```python
from build123d import *

# Parameters (mm, degrees)
BOSS_EXTRUDE1_DEPTH     = 152.4
CUT_EXTRUDE1_DEPTH      = 1634.518215387
CUT_EXTRUDE1_DEPTH_BACK = 1634.518215387
CUT_EXTRUDE2_DEPTH      = 1634.518215536
FILLET1_R               = 50.8
CUT_EXTRUDE3_DEPTH      = 48.26
CUT_EXTRUDE4_DEPTH      = 1213.010253568
SKETCH6_W               = 101.6
SKETCH6_H               = 127
CUT_EXTRUDE5_DEPTH      = 25.4
LPATTERN1_COUNT         = 2
LPATTERN1_PITCH         = 254
SKETCH7_W               = 304.8
SKETCH7_H               = 127
CUT_EXTRUDE7_DEPTH      = 114.3


with BuildPart() as part:
    # Sketch1 → Boss-Extrude1 (new body)
    with BuildSketch(Plane.XY):
        with BuildLine():
            Line((0, 0), (0, 381))
            Line((0, 381), (457.2, 1016))
            Line((457.2, 1016), (1270, 1016))
            Line((1270, 1016), (1270, 381))
            ThreePointArc((1270, 381), (1000.592316368, 269.407683632), (889, 0))
            Line((889, 0), (0, 0))
        make_face()
    extrude(amount=BOSS_EXTRUDE1_DEPTH)

    # Sketch3 → Cut-Extrude1 (cut, two sides: drawn at the far end of the back side and taken through both)
    with BuildSketch(Plane(origin=(1270, 0, 0), x_dir=(0, 0, -1), z_dir=(1, 0, 0)).offset(-CUT_EXTRUDE1_DEPTH_BACK)):
        with BuildLine():
            Line((0, 1016), (-114.3, 1016))
            add(Edge.make_bspline(
                [(-114.3, 1016), (-8.40924149, 829.104015067), (-15.870449407, 600.128785321), (0, 381)],
                knots=[0, 0, 0, 0, 1, 1, 1, 1], degree=3))
            Line((0, 381), (0, 1016))
        make_face()
    extrude(amount=CUT_EXTRUDE1_DEPTH + CUT_EXTRUDE1_DEPTH_BACK, mode=Mode.SUBTRACT)

    # Sketch4 → Cut-Extrude2 (cut, through all)
    with BuildSketch(Plane.ZY):
        with BuildLine():
            Line((0, 0), (63.5, 0))
            add(Edge.make_bspline(
                [(0, 381), (19.94820776, 253.802921476), (11.059212426, 124.818838522), (63.5, 0)],
                knots=[0, 0, 0, 0, 1, 1, 1, 1], degree=3))
            Line((0, 381), (0, 0))
        make_face()
    extrude(amount=-CUT_EXTRUDE2_DEPTH, mode=Mode.SUBTRACT)

    # Fillet1
    fillet1_edges = [part.edges().sort_by_distance(p)[0] for p in [
        (635, 381, 0),
    ]]
    fillet(fillet1_edges, radius=FILLET1_R)

    # Sketch5 → Cut-Extrude3 (cut)
    with BuildSketch(Plane.XY.offset(152.4)):
        Polygon((1186.404527601, 953.507993358), (1186.404527601, 470.907993358), (149.686717373, 470.907993358), (475.204527601, 953.507993358), align=None)
    extrude(amount=-CUT_EXTRUDE3_DEPTH, mode=Mode.SUBTRACT)

    # 3DSketch1 → Cut-Extrude4 (cut, through all)
    with BuildSketch(Plane(origin=(491.411031078, 923.027993358, 104.14), x_dir=(0.8443699387246085, -0.535760586995909, 0), z_dir=(0, 0, -1))):
        Polygon((0, 0), (-14.240523347, 508.390329239), (786.993314242, 0), (561.095220341, -356.020140964), align=None)
    extrude(amount=CUT_EXTRUDE4_DEPTH, mode=Mode.SUBTRACT)

    # Sketch6 → Cut-Extrude5 (cut)
    with BuildSketch(Plane(origin=(-180.663856691, 130.077976818, 0), x_dir=(0, 0, 1), z_dir=(-0.8115343414514944, 0.5843047258450759, 0))):
        with Locations((101.6, 448.894584093)):
            Rectangle(SKETCH6_W, SKETCH6_H)
    cut_extrude5 = extrude(amount=-CUT_EXTRUDE5_DEPTH, mode=Mode.SUBTRACT)

    # LPattern1: Cut-Extrude5 ×2
    with Locations(*[Vector(0.5843047258450758, 0.8115343414514946, 0) * (i * LPATTERN1_PITCH) for i in range(1, LPATTERN1_COUNT)]):
        add(cut_extrude5, mode=Mode.SUBTRACT)

    # Sketch7 → Cut-Extrude7 (cut)
    with BuildSketch(Plane.XY.offset(-16.17222699)):
        with Locations((800.1, 359.431211457)):
            Rectangle(SKETCH7_W, SKETCH7_H)
    extrude(amount=CUT_EXTRUDE7_DEPTH, mode=Mode.SUBTRACT)


solid = part.part
```
Verification items for the finished model (mm, model axes). A direction names the side the tool comes from. Give positions to 0.01 mm unless a question says otherwise; leave off trailing zeros. Order: outer loops, then holes, each group sorted by start corner. A loop starts at its lowest first (then second) coordinate and runs counter-clockwise, first axis right, second up. Notation, with made-up numbers: M 2.25,-1.5 L 8.25,-1.5 A16 cw 8.25,7.5 Z; hole C 69,-10 d6. An arc over 180 degrees is marked long. Answer in a Markdown table with one row per item. Add a question column.
Item 1: Tool access check on faces 1 (the flat face through (675, 501.388, 56)), 2 (the flat face through (952.5, 359, 49)), 3 (the flat face through (1186.405, 716, 129)). Record the directions out of +Z, -Z, +X, -X, +Y, -Y that give a thin tool (end or side, any length) a straight path to the whole face; none if there is none.
Item 2: Mould release check, pull along X, two halves, no side actions. Record for faces 4 (the flat face through (858, 1016, 133)), 5 (the flat face through (747, 499, 104.14)), 6 (the flat face through (174.6, 623.5, 92.2)): released by +X, released by -X, zero draft, split by the parting line, or undercut.
Item 3: Gauge pin test, flat ends, axial feed: pin 1 (1.5 mm diameter, centred on x = 752, z = 33.5, fed in from +Y); pin 2 (14.5 mm diameter, centred on y = 693.5, z = 131.5, fed in from -X); pin 3 (24 mm diameter, centred on x = 950.5, z = 136.5, fed in from -Y). Record the tip position at first contact, or that the pin passes through.
Item 4: Section check A-A, the plane z = 131. Enter the section's corners in (x, y), and give its area (3 significant figures).
Item 5: Scan lines: probe 1 along Y at (x, z) = (624.5, 119); probe 2 along X at (y, z) = (648.5, 89.5); probe 3 along Y at (x, z) = (919, 141). Record each from-to range of solid material in increasing order. Write a range as from..to.
Filled sheet:
| question | item | result |
|---|---|---|
| 1 | face 1 | +Z, -Z |
| 1 | face 2 | -Z |
| 1 | face 3 | +Z |
| 2 | face 4 | zero draft |
| 2 | face 5 | undercut |
| 2 | face 6 | released by -X |
| 3 | pin 1 | stops at y = 501.39 |
| 3 | pin 2 | stops at x = 251.08 |
| 3 | pin 3 | stops at y = 187.8 |
| 4 | outline | M 0,0 L 889,0 A381 cw 1270,381 L 1270,1016 L 457.2,1016 L 267.14,752.03 L 287.76,737.19 L 213.55,634.13 L 192.94,648.97 L 118.73,545.9 L 139.34,531.06 L 65.14,428 L 44.52,442.84 L 0,381 Z; hole M 149.69,470.91 L 1186.4,470.91 L 1186.4,953.51 L 475.2,953.51 Z |
| 4 | area | 603,000 mm^2 |
| 5 | probe 1 | y = 0..470.91, 953.51..1016 |
| 5 | probe 2 | x = 192.6..193.59, 223.9..306.24, 1155.92..1270 |
| 5 | probe 3 | y = 148.19..470.91, 953.51..1016 |
